Design review of the part built by this model. Coordinates are the model's own, in mm. A direction names the side the tool comes from. Coordinates: 2 decimals unless noted, no trailing zeros.
Q1. To check wall thickness, follow probe 1 along X at (y, z) = (-4.5, 13); probe 2 along X at (y, z) = (-0.75, 17); probe 3 along Z at (x, y) = (35.5, -2). State the ranges of each line that lie inside material, in increasing order.
Q2. Machinability: for faces 1 (the face through (-46, -4, 43.947)), 2 (the face through (-31.79, -3.51, 41.26)), 3 (the face through (-34.67, -3.51, 3.47)), which of the approach directions +Z, -Z, +X, -X, +Y, -Y give a long, thin tool a straight path to every point of the face, cutting with its end or side? Answer none if there is none.
Q3. The part is to be moulded in two halves that separate along Z. For faces 4 (the face through (7.041, -3.506, 43.785)), 5 (the face through (62.276, -3.506, 5.843)), 6 (the face through (61.57, -3.51, 12.32)), say which applies: +Z half, -Z half, draft (parallel to the pull), parting line (faces both ways), or undercut.
Q4. Clearance check with flat-ended pins moving along their axes: pin 1 Ø2 at (y, z) = (-2.5, 11.5) entering from -X; pin 2 Ø1.5 at (x, y) = (-85, -5) entering from +Z; pin 3 Ø4 at (x, y) = (41, -1.5) entering from +Z. State where each tip first meets the part, or that it passes through.
from build123d import *

# Parameters (mm, degrees)
F0_R     = 11.1002676346
F1_DEPTH = 7.112


with BuildPart() as f1:
    # F0 (on Front) → F1 (new body)
    with BuildSketch(Plane.XZ):
        with BuildLine():
            ThreePointArc((-28.9238487713, 43.4874370513), (-31.8417154654, 41.2631470908), (-34.3433879316, 43.9469963312))
            Line((-34.3433879316, 43.9469963312), (-38.5404489934, 43.9469963312))
            ThreePointArc((-38.5404489934, 43.9469963312), (-41.1935001612, 41.8414797087), (-43.8465513289, 43.9469963312))
            Line((-43.8465513289, 43.9469963312), (-47.7376915514, 43.9469963312))
            ThreePointArc((-47.7376915514, 43.9469963312), (-50.4202209413, 41.6067623115), (-53.1027503312, 43.9469963312))
            Line((-53.1027503312, 43.9469963312), (-57.0200905204, 43.7591150403))
            ThreePointArc((-57.0200905204, 43.7591150403), (-57.0113369766, 43.092435836), (-57.1736224025, 42.4457510391))
            ThreePointArc((-57.1736224025, 42.4457510391), (-60.0285652732, 40.8507993338), (-62.1561594307, 43.3343276381))
            add(Edge.make_bspline(
                [(-112.0357811451, 23.9776968956), (-92.9390639067, 36.2371653318), (-71.5056391184, 42.7196059605), (-62.1561594307, 43.3343276381)],
                knots=[0, 0, 0, 0, 0.7368858585, 0.7368858585, 0.7368858585, 0.7368858585], degree=3))
            add(Edge.make_bspline(
                [(-36.7892459035, 0.9486632771), (-66.7406320572, 2.1232275758), (-95.9974229336, 3.8856838364), (-112.0357811451, 23.9776968956)],
                knots=[0, 0, 0, 0, 78.6916606463, 78.6916606463, 78.6916606463, 78.6916606463], degree=3))
            Line((-36.7892459035, 0.9486632771), (-32.4876937115, 6.072126331))
            ThreePointArc((-32.4876937115, 6.072126331), (-32.6386039848, 19.4193686965), (-19.6879729629, 22.6524490863))
            ThreePointArc((-19.6879729629, 22.6524490863), (-18.3323991504, 21.9194060304), (-17.0953891825, 21.0003092879))
            add(Edge.make_bspline(
                [(6.6555179041, 19.1500785461), (0.9244663771, 17.9030998445), (-10.7726783896, 18.050524278), (-17.0953891825, 21.0003092879)],
                knots=[0, 0, 0, 0, 0.49185709, 0.49185709, 0.49185709, 0.49185709], degree=3))
            add(Edge.make_bspline(
                [(36.9700267911, 11.1494921148), (32.886029432, 16.2799953356), (27.8643252538, 23.8588869819), (11.8520011969, 20.5491422263), (6.6555179041, 19.1500785461)],
                knots=[0, 0, 0, 0, 0.3035047621, 0.4422302713, 0.4422302713, 0.4422302713, 0.4422302713], degree=3))
            ThreePointArc((36.9700267911, 11.1494921148), (62.5770277208, 6.1588707444), (55.6138120592, 31.3012339175))
            add(Edge.make_bspline(
                [(25.7371558529, 42.729893316), (34.6145431232, 35.8809284759), (45.6531612823, 35.1182930171), (55.6138120592, 31.3012339175)],
                knots=[0, 0, 0, 0, 31.9879483824, 31.9879483824, 31.9879483824, 31.9879483824], degree=3))
            Line((25.7371558529, 42.729893316), (-12.1854665813, 44.8704426206))
            add(Edge.make_bspline(
                [(-12.1854665813, 44.8704426206), (-20.3191175134, 42.9574390185), (-28.4139272796, 42.8222121718), (-28.9238487713, 43.4874370513)],
                knots=[0.0361898776, 0.0361898776, 0.0361898776, 0.0361898776, 0.7742766932, 0.7742766932, 0.7742766932, 0.7742766932], degree=3))
        make_face()
        with Locations((51.3174180221, 16.575922902)):
            Circle(F0_R, mode=Mode.SUBTRACT)
    extrude(amount=F1_DEPTH)


solid = f1.part
Here are the results:
1. probe 1: x = -99.35 to -34.88, 35.51 to 40.81, 61.83 to 66.23
1. probe 2: x = -105.1 to -34.05, 32.01 to 40.23, 62.41 to 66.65
1. probe 3: z = 13.01 to 37.46
2. face 1: +Z, -X, +Y, -Y
2. face 2: +Z, +Y, -Y
2. face 3: -Z, +Y, -Y
3. face 4: +Z half
3. face 5: parting line
3. face 6: undercut
4. pin 1: stops at x = -98.49
4. pin 2: stops at z = 37.73
4. pin 3: stops at z = 36.27
